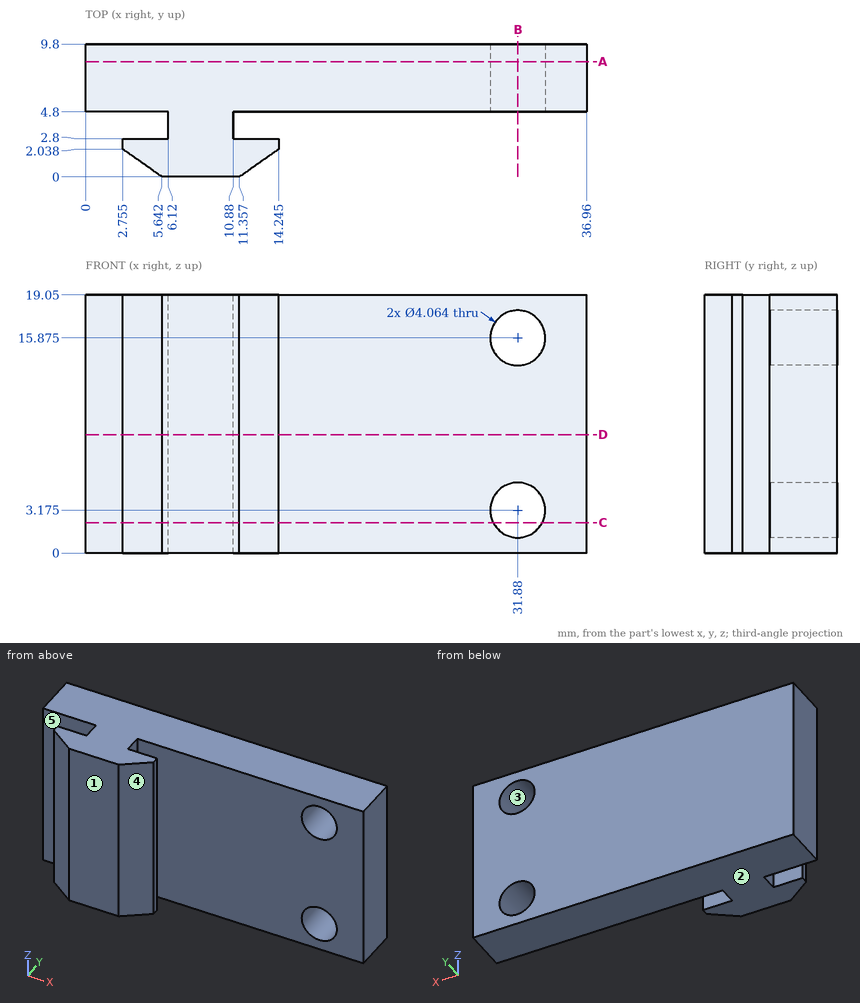
Source: three-view drawing plus pictorial views. Frame: mm from the lowest corner of the part. A direction names the side the tool comes from. Round coordinates to 2 decimals unless told otherwise and drop trailing zeros. Order: outer loops, then holes, each group sorted by start corner. A loop starts at its lowest first (then second) coordinate and runs counter-clockwise, first axis right, second up. Notation, with made-up numbers: (-36.5, -17) -> (-19.5, -17) arc R7 ccw to (-19.5, -7) -> close; hole circle Ø10 at (89, 52.25). An arc over 180 degrees is marked (long way). Use CSV: the item, a comma, the result in double quotes. Start each with the question number.
1) Section A-A (y = 8.5). State how many separate pieces and enclosed holes the cut face has, and give its area (3 significant figures).
2) Section C-C (z = 2.25). Return the cut outline in (x, y) (1 decimal).
3) Draft query along Z for the marked faces 1, 2 and 3. Return one class per face: +Z half, -Z half, draft (parallel to the pull), parting line (faces both ways), or undercut.
4) Material intervals for line 1 along Z through (x, y) = (31.88, 7.65); line 2 along Y through (x, z) = (6, 2.25); line 3 along X through (y, z) = (2.75, 13.5) (1 decimal), sorted ascending. Write a range as from..to.
5) Set-up query: the marked faces 4 and 5. Return all of +Z, -Z, +X, -X, +Y, -Y with unobstructed straight access to the full face (end or side cutting, diameter ignored); none if empty.
6) Section B-B (x = 31.88). Return the cut outline in (y, z).
7) First-contact query: pin 1 Ø1.8 at (x, z) = (2, 10.5) entering from -Y (1 decimal); pin 2 Ø5.5 at (x, z) = (31.88, 15.875) entering from -Y; pin 3 Ø0.6 at (y, z) = (2.5, 12) entering from +X (1 decimal). Flat tips, straight axial feed; report the tip coordinate or a pass-through.
8) Section D-D (z = 8.75). Return the cut outline in (x, y) (1 decimal), and give its area (3 significant figures).
Returned:
1,separate pieces,"1"
1,enclosed holes,"2"
1,area,"678 mm²"
2,outline,"(0, 4.8) -> (6.1, 4.8) -> (6.1, 2.8) -> (2.8, 2.8) -> (2.8, 2) -> (5.6, 0) -> (11.4, 0) -> (14.2, 2) -> (14.2, 2.8) -> (10.9, 2.8) -> (10.9, 4.8) -> (30.1, 4.8) -> (30.1, 9.8) -> (0, 9.8) -> close; (33.7, 4.8) -> (37, 4.8) -> (37, 9.8) -> (33.7, 9.8) -> close"
3,face 1,"draft"
3,face 2,"-Z half"
3,face 3,"undercut"
4,line 1,"z = 0..1.14, 5.21..13.84, 17.91..19.05"
4,line 2,"y = 0..2.8, 4.8..9.8"
4,line 3,"x = 2.8..14.2"
5,face 4,"+Z, -Z, +X, -Y"
5,face 5,"+Z, -Z, -X"
6,outline,"(4.8, 0) -> (9.8, 0) -> (9.8, 1.14) -> (4.8, 1.14) -> close; (4.8, 5.21) -> (9.8, 5.21) -> (9.8, 13.84) -> (4.8, 13.84) -> close; (4.8, 17.91) -> (9.8, 17.91) -> (9.8, 19.05) -> (4.8, 19.05) -> close"
7,pin 1,"stops at y = 1.9"
7,pin 2,"stops at y = 4.8"
7,pin 3,"stops at x = 14.2"
8,outline,"(0, 4.8) -> (6.1, 4.8) -> (6.1, 2.8) -> (2.8, 2.8) -> (2.8, 2) -> (5.6, 0) -> (11.4, 0) -> (14.2, 2) -> (14.2, 2.8) -> (10.9, 2.8) -> (10.9, 4.8) -> (37, 4.8) -> (37, 9.8) -> (0, 9.8) -> close"
8,area,"221 mm²"
